from build123d import *

# Parameters (mm, degrees)
F0_R     = 7
F1_DEPTH = 21.5
F2_R     = 5.5
F3_DEPTH = 43.001
F2_R_2   = 7
F4_DEPTH = 19


with BuildPart() as f1:
    # F0 (on Front) → F1 (new body, symmetric)
    with BuildSketch(Plane.XZ):
        with BuildLine():
            Line((-7, 18), (-14, 11))
            Line((-14, 11), (-14, -7))
            Line((-14, -7), (-7, -14))
            Line((-7, -14), (21.0666262554, -14))
            ThreePointArc((21.0666262554, -14), (24.3318620364, -15.2134137678), (26.0122649968, -18.2647058824))
            ThreePointArc((26.0122649968, -18.2647058824), (28.3490951999, -26.115672061), (32.7880673968, -33))
            Line((32.7880673968, -33), (38, -33))
            Line((38, -33), (67, 0))
            Line((67, 0), (67, 19))
            Line((67, 19), (62, 24))
            Line((62, 24), (38, 24))
            ThreePointArc((38, 24), (29.5749729609, 16.2760691513), (18.2430849879, 14.7832519053))
            Line((18.2430849879, 14.7832519053), (0, 18))
            Line((0, 18), (-7, 18))
        make_face()
        Circle(F0_R, mode=Mode.SUBTRACT)
    extrude(amount=F1_DEPTH, both=True)

    # F2 (on face) → F3 (cut, through all)
    with BuildSketch(Plane.XZ.offset(21.5)):
        with Locations((53, 10)):
            Circle(F2_R)
    extrude(amount=-F3_DEPTH, mode=Mode.SUBTRACT)

    # F2 (on face) → F4 (cut)
    with BuildSketch(Plane.XZ.offset(21.5)):
        Polygon((15, -14), (15, 15.3550952894), (0, 18), (-7, 18), (-14, 11), (-14, -7), (-7, -14), align=None)
        Circle(F2_R_2, mode=Mode.SUBTRACT)
    extrude(amount=-F4_DEPTH, mode=Mode.SUBTRACT)


solid = f1.part
Can you work these out from the model? Positions are in its coordinate system, mm. A direction names the side the tool comes from. Round coordinates to 2 decimals unless told otherwise and drop trailing zeros. Write each loop counter-clockwise with the first axis right and the second up, starting at its lowest first coordinate (ties: lowest second). Pieces come first, ordered by that corner, then holes. Notation, with made-up numbers: M -21,65 L 2,65 A25 ccw 2,78 Z; hole C 37,31 d11. An arc over 180 degrees is marked long. Use CSV: the item, a comma, the result in double quotes.
(1) On a 3-axis mill with a long thin cutter (end or side, diameter ignored), from which of +Z, -Z, +X, -X, +Y, -Y can I reach the whole of each face in a straight line? I mean faces 1 (the flat face through (10, 4, -14)), 2 (the flat face through (11.28, 4.48, 16.01)), 3 (the flat face through (7, -2.5, 2)). Say none if no direction works.
Check values:
face 1,"-Z, -X, +Y, -Y"
face 2,"+Z, +Y, -Y"
face 3,"+Z, -Z, -X, -Y"
(2) Imagine slicing it at A-A (y = -6). Write out the boundary of the cut face in (x, z).
Check values:
outline,"M 15,-14 L 21.07,-14 A5 cw 26.01,-18.26 A29 ccw 32.79,-33 L 38,-33 L 67,0 L 67,19 L 62,24 L 38,24 A19 cw 18.24,14.78 L 15,15.36 Z; hole C 53,10 d11"
(3) We'd pull the mould along Z, two halves only. Please class faces 4 (the cylindrical face through (47.505, -0.301, 10.242)), 5 (the flat face through (41, -21.5, 2)), 6 (the flat face through (-10, 9, 15)), 7 (the cylindrical face through (6.466, 9.668, -2.681)): +Z half, -Z half, draft (parallel to the pull), parting line (faces both ways), or undercut.
Check values:
face 4,"undercut"
face 5,"draft"
face 6,"+Z half"
face 7,"undercut"
(4) Imagine slicing it at C-C (x = 53). Write out the boundary of the cut face in (y, z).
Check values:
outline,"M -21.5,-15.93 L 21.5,-15.93 L 21.5,4.5 L -21.5,4.5 Z; M -21.5,15.5 L 21.5,15.5 L 21.5,24 L -21.5,24 Z"
(5) I'm going to push flat-ended pins straight in: pin 1 (9 mm diameter, centred on x = 53, z = 10, fed in from -Y); pin 2 (5.5 mm diameter, centred on x = -3, y = 9.5, fed in from +Z); pin 3 (1 mm diameter, centred on y = -13.5, z = -26.5, fed in from +X); pin 4 (8.5 mm diameter, centred on x = -2.5, z = 5, fed in from -Y). Where does each tip first touch, or does it pass through?
Check values:
pin 1,"through"
pin 2,"z = 18"
pin 3,"x = 44.15"
pin 4,"y = -2.5"
(6) I need wall thicknesses on line 1 along Z through (x, y) = (0, 16); line 2 along X through (y, z) = (16, 0.5); line 3 along Y through (x, z) = (-4.5, 13.5). Which ranges of each line are inside material? Lowest first, please.
Check values:
line 1,"-14 to -7, 7 to 18"
line 2,"-14 to -6.98, 6.98 to 67"
line 3,"-2.5 to 21.5"
(7) Imagine slicing it at B-B (z = 10). Write out the boundary of the cut face in (x, y), plus the area to 3 significant figures.
Check values:
outline,"M -14,-2.5 L 15,-2.5 L 15,-21.5 L 47.5,-21.5 L 47.5,21.5 L -14,21.5 Z; M 58.5,-21.5 L 67,-21.5 L 67,21.5 L 58.5,21.5 Z"
area,"2,460 mm^2"
(8) Imagine slicing it at D-D (y = 14.5). Write out the boundary of the cut face in (x, z), plus the area to 3 significant figures.
Check values:
outline,"M -14,-7 L -7,-14 L 21.07,-14 A5 cw 26.01,-18.26 A29 ccw 32.79,-33 L 38,-33 L 67,0 L 67,19 L 62,24 L 38,24 A19 cw 18.24,14.78 L 0,18 L -7,18 L -14,11 Z; hole C 0,0 d14; hole C 53,10 d11"
area,"2,670 mm^2"
